Geometry check sheet. Reference: the model listing, model coordinates, mm. Face numbers are marked on the shaded views. Coordinates: 2 decimals unless noted, no trailing zeros. Loops run counter-clockwise (first coordinate to the right, second up) from the corner with the lowest first, then second, coordinate; pieces in that order, holes last.
from build123d import *

# Parameters (mm, degrees)
SKETCH1_R           = 7.5
SKETCH1_R_2         = 0.75
BOSS_EXTRUDE1_DEPTH = 20
CHAMFER1_SIZE       = 6
CHAMFER1_SIZE2      = 16.484864517
SKETCH2_R           = 3.5
CUT_EXTRUDE1_DEPTH  = 3


with BuildPart() as part:
    # Sketch1 → Boss-Extrude1 (new body)
    with BuildSketch(Plane(origin=(0, 0, 0), x_dir=(1, 0, 0), z_dir=(0, 1, 0))):
        with Locations(Location((0, 0, 0), (0, 0, 270))):
            Circle(SKETCH1_R)
        with Locations(Location((0, 0, 0), (0, 0, 270))):
            Circle(SKETCH1_R_2, mode=Mode.SUBTRACT)
    extrude(amount=BOSS_EXTRUDE1_DEPTH)

    # Chamfer1
    chamfer1_edges = [part.edges().sort_by_distance(p)[0] for p in [
        (0, 20, -0.75),
    ]]
    chamfer1_side = [part.faces().sort_by_distance(p)[0] for p in [
        (0, 20, -7.287867966),
    ]]
    chamfer(chamfer1_edges, length=CHAMFER1_SIZE, length2=CHAMFER1_SIZE2, reference=chamfer1_side[0])

    # Sketch2 → Cut-Extrude1 (cut)
    with BuildSketch(Plane.XZ):
        with Locations((0, 5)):
            Circle(SKETCH2_R)
    extrude(amount=-CUT_EXTRUDE1_DEPTH, mode=Mode.SUBTRACT)


solid = part.part
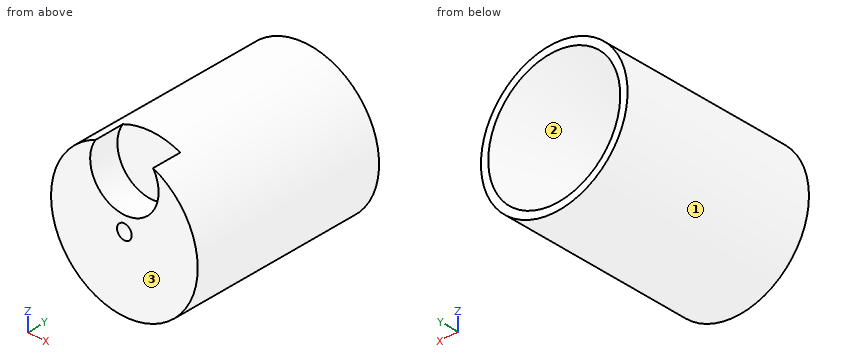
1) Section check A-A on x = 0. Record the cut outline in (y, z).
Data:
outline: (0, -7.5) - (20, -7.5) - (20, -6.75) - (3.52, -0.75) - (0, -0.75) - close; (0, 0.75) - (3.52, 0.75) - (20, 6.75) - (20, 7.5) - (3, 7.5) - (3, 1.5) - (0, 1.5) - close
2) Material ranges on probe 1 along X at (y, z) = (2.25, 0); probe 2 along X at (y, z) = (2.5, 2.5); probe 3 along Z at (x, y) = (-5, 18.75), recorded low to high.
Data:
probe 1: x = -7.5 to -0.75, 0.75 to 7.5
probe 2: x = -7.07 to -2.45, 2.45 to 7.07
probe 3: z = -5.59 to -3.82, 3.82 to 5.59
3) Mould release check, pull along X, two halves, no side actions. Record for the marked faces 1, 2 and 3: +X half, -X half, draft (parallel to the pull), parting line (faces both ways), or undercut.
Data:
face 1: parting line
face 2: undercut
face 3: draft
4) Section check C-C on y = 8.25. Record the cut outline in (x, z).
Data:
outline: circle Ø15 at (0, 0); hole circle Ø4.95 at (0, 0)
5) Section check B-B on z = 0. Record the cut outline in (x, y).
Data:
outline: (-7.5, 0) - (-0.75, 0) - (-0.75, 3.52) - (-6.75, 20) - (-7.5, 20) - close; (0.75, 0) - (7.5, 0) - (7.5, 20) - (6.75, 20) - (0.75, 3.52) - close
6) Section check D-D on y = 14.75. Record the cut outline in (x, z), and give its area (3 significant figures).
Data:
outline: circle Ø15 at (0, 0); hole circle Ø9.68 at (0, 0)
area: 103 mm2
7) Depth check by flat-ended pin: pin 1 (1.8 mm diameter, centred on x = 0.5, z = 4, fed in from -Y); pin 2 (1.5 mm diameter, centred on x = -1.5, y = 14.5, fed in from +Z). Enter the tip coordinate at first touch or a pass-through.
Data:
pin 1: stops at y = 3
pin 2: stops at z = 7.46
